from build123d import *

# Parameters (mm, degrees)
SKETCH_2_R          = 6
CUT_EXTRUDE_1_DEPTH = 27
CUT_EXTRUDE_2_DEPTH = 4
CHAMFER_2_SIZE      = 2
CHAMFER_3_SIZE      = 1
CHAMFER_4_SIZE      = 0.5
CUT_EXTRUDE_3_DEPTH = 10


with BuildPart() as part:
    # 草图1 → 旋转1 (revolve)
    with BuildSketch(Plane.XY):
        Polygon((0, 0), (9, 0), (9, 15), (8, 15), (8, 16), (8, 16.5), (10, 16.5), (10, 16), (13, 16), (13, 17), (15, 17), (15, 26), (0, 26), align=None)
    revolve(axis=Axis((0, 26, 0), (0, -1, 0)))

    # 草图2 → 切除-拉伸1 (cut, through all)
    with BuildSketch(Plane.XZ):
        Circle(SKETCH_2_R)
    extrude(amount=-CUT_EXTRUDE_1_DEPTH, mode=Mode.SUBTRACT)

    # 草图3 → 切除-拉伸2 (cut)
    with BuildSketch(Plane(origin=(0, 26, 0), x_dir=(1, 0, 0), z_dir=(0, 1, 0))):
        with BuildLine():
            Line((11, 10.198039027), (11, -10.198039027))
            ThreePointArc((11, -10.198039027), (15, 0), (11, 10.198039027))
        make_face()
    extrude(amount=-CUT_EXTRUDE_2_DEPTH, mode=Mode.SUBTRACT)

    # 倒角2
    chamfer_2_edges = [part.edges().sort_by_distance(p)[0] for p in [
        (-6, 26, 0),
    ]]
    chamfer(chamfer_2_edges, length=CHAMFER_2_SIZE)

    # 倒角3
    chamfer_3_edges = [part.edges().sort_by_distance(p)[0] for p in [
        (-9, 0, 0),
        (-15, 17, 0),
        (-15, 26, 0),
    ]]
    chamfer(chamfer_3_edges, length=CHAMFER_3_SIZE)

    # 倒角4
    chamfer_4_edges = [part.edges().sort_by_distance(p)[0] for p in [
        (-9, 15, 0),
        (-6, 0, 0),
    ]]
    chamfer(chamfer_4_edges, length=CHAMFER_4_SIZE)

    # 草图4 → 切除-拉伸3 (cut)
    with BuildSketch(Plane(origin=(0, 26, 0), x_dir=(1, 0, 0), z_dir=(0, 1, 0))):
        with BuildLine():
            Line((3.161317604, -14.663085317), (14.86002737, 2.044403717))
            ThreePointArc((14.86002737, 2.044403717), (14.305754261, -4.510586993), (11, -10.198039027))
            ThreePointArc((11, -10.198039027), (7.424276979, -13.033806479), (3.161317604, -14.663085317))
        make_face()
    extrude(amount=-CUT_EXTRUDE_3_DEPTH, mode=Mode.SUBTRACT)


solid = part.part
Part model, mm, in its own coordinate system. A direction names the side the tool comes from. Coordinates: 2 decimals unless noted, no trailing zeros. Loops run counter-clockwise (first coordinate to the right, second up) from the corner with the lowest first, then second, coordinate; pieces in that order, holes last. Notation, with made-up numbers: (70.25, -30) -> (95.25, -30) arc R19 ccw to (95.25, -8) -> close; hole circle Ø9 at (85, 48). An arc over 180 degrees is marked (long way). Use a Markdown table: item, result. Add a question column.
Item 1: Band-saw the part on A-A on y = 7.5. Write the cut outline in (x, z), plus the area to 3 significant figures.
Item 2: Pull direction X, two halves, no side cores. Call faces 1 (the flat face through (0, 16.5, 8.2)), 2 (the conical face through (-13.641, 25.826, -3.85)), 3 (the flat face through (11, 24, -3)): +X half, -X half, draft (parallel to the pull), parting line (faces both ways), or undercut.
Item 3: Band-saw the part on B-B on y = 15.5. Write the cut outline in (x, z).
Item 4: Probe probe 1 along Z at (x, y) = (0, 9.5); probe 2 along Y at (x, z) = (-2.5, -9.5); probe 3 along Y at (x, z) = (10.25, 2). List the from-to ranges inside material, lowest first.
Item 5: Flat gauge pins, fed straight in: P1, Ø6, axis at x = 7.5, z = 0.5, coming from the -Y side; P2, Ø2, axis at x = -2, z = -9, coming from the -Y side; P3, Ø1.5, axis at x = -6, y = 8.5, coming from the +Z side; P4, Ø10, axis at y = 16, z = 10.5, coming from the +X side. Where does each tip first touch, or does it go through?
Item 6: Which spindle directions (+Z, -Z, +X, -X, +Y, -Y) get a long thin tool onto all of the face, cutting with end or side? Do faces 4 (the cylindrical face through (-1.73, 15.76, -7.81)), 5 (the flat face through (12, 22, -3)), 6 (the flat face through (-8, 16, -7)), 7 (the flat face through (-7, 26, -6)), 8 (the cylindrical face through (-6, 12, 0)). Say none if no direction does.
Geometry says:
| question | item | result |
|---|---|---|
| 1 | outline | circle Ø18 at (0, 0); hole circle Ø12 at (0, 0) |
| 1 | area | 141 mm² |
| 2 | face 1 | undercut |
| 2 | face 2 | parting line |
| 2 | face 3 | +X half |
| 3 | outline | circle Ø16 at (0, 0); hole circle Ø12 at (0, 0) |
| 4 | probe 1 | -9 to -6, 6 to 9 |
| 4 | probe 2 | 16.5 to 26 |
| 4 | probe 3 | 16 to 26 |
| 5 | P1 | y = 0 |
| 5 | P2 | y = 0.22 |
| 5 | P3 | z = 7.31 |
| 5 | P4 | x = 9.58 |
| 6 | face 4 | none |
| 6 | face 5 | +Z, -Z, +X, +Y |
| 6 | face 6 | -Y |
| 6 | face 7 | +Z, -Z, +X, -X, +Y |
| 6 | face 8 | +Y, -Y |
